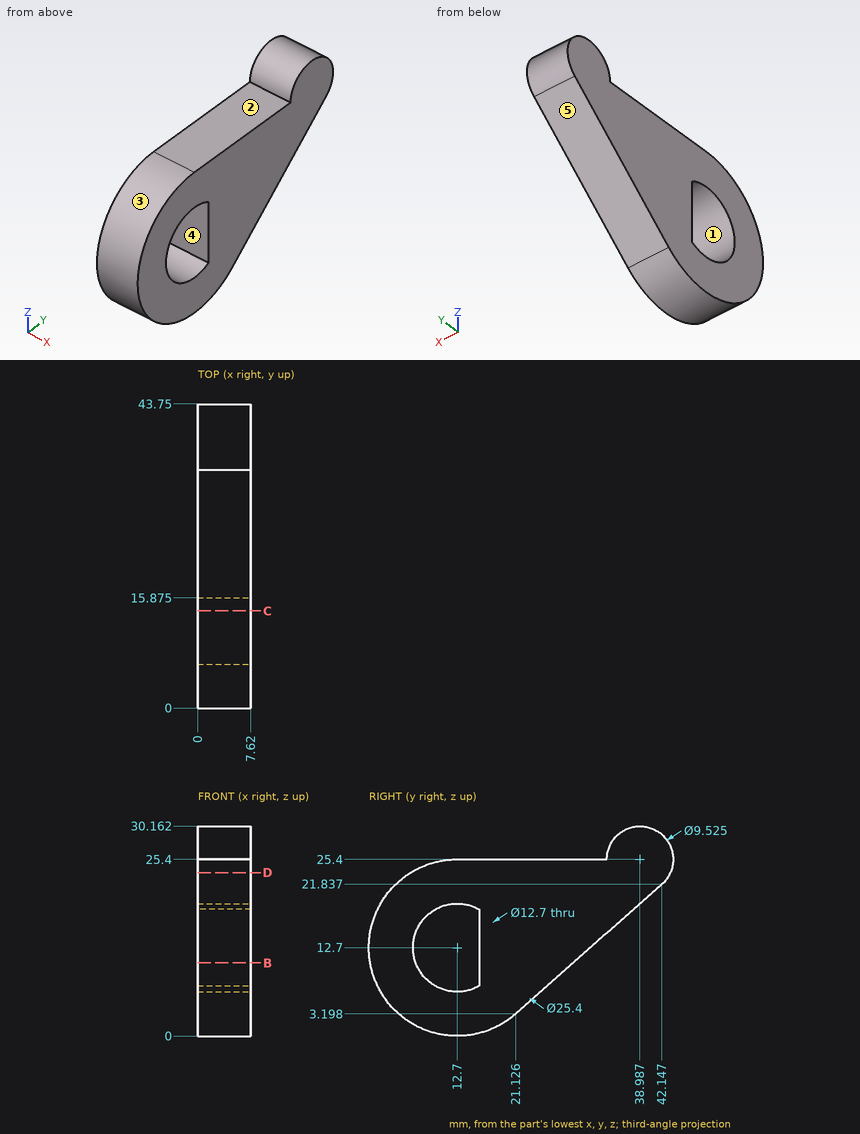
Part print with two shaded views. Sizes in mm from the minimum x, y, z corner. A direction names the side the tool comes from. Round coordinates to 2 decimals unless told otherwise and drop trailing zeros. Order: outer loops, then holes, each group sorted by start corner. A loop starts at its lowest first (then second) coordinate and runs counter-clockwise, first axis right, second up. Notation, with made-up numbers: (60.25, 78) - (80.25, 78) arc R28 ccw to (80.25, 98) - close; hole circle Ø10 at (55, -16). An arc over 180 degrees is marked (long way). Answer in a Markdown table with one row per item. Add a question column.
(1) Mould opens along Z. For the marked faces 3, 4 and 5 say: +Z half, -Z half, draft (parallel to the pull), parting line (faces both ways), or undercut.
(2) Band-saw the part on B-B on z = 10.5. List the corners of the cut face in (x, y) (1 decimal), and give its area (3 significant figures).
(3) Band-saw the part on C-C on y = 14. List the corners of the cut face in (x, z) (1 decimal).
(4) Band-saw the part on D-D on z = 23.5. List the corners of the cut face in (x, y) (1 decimal).
(5) 3-axis set-ups, long thin cutter, end or side, ignore diameter. For the marked faces 1 and 2: which of +Z, -Z, +X, -X, +Y, -Y reach the whole face in a straight line?
(6) Probe L1, parallel to Z at x = 2.5, y = 12.7; L2, parallel to Z at x = 4.5, y = 14 (1 decimal); L3, parallel to Y at x = 1.5, z = 13.5 (1 decimal). List the from-to ranges inside material, lowest first. Write a range as [from, to].
(7) Drop flat-ended pins along their axis: pin 1 Ø3 at (x, y) = (2, 19) entering from +Z; pin 2 Ø2 at (x, y) = (6, 6) entering from -Z. Give the stop position or say it passes through.
Data:
| question | item | result |
|---|---|---|
| 1 | face 3 | parting line |
| 1 | face 4 | undercut |
| 1 | face 5 | -Z half |
| 2 | outline | (0, 0.2) - (7.6, 0.2) - (7.6, 6.7) - (0, 6.7) - close; (0, 15.9) - (7.6, 15.9) - (7.6, 29.4) - (0, 29.4) - close |
| 2 | area | 153 mm^2 |
| 3 | outline | (0, 0.1) - (7.6, 0.1) - (7.6, 6.5) - (0, 6.5) - close; (0, 18.9) - (7.6, 18.9) - (7.6, 25.4) - (0, 25.4) - close |
| 4 | outline | (0, 6) - (7.6, 6) - (7.6, 43.4) - (0, 43.4) - close |
| 5 | face 1 | +X, -X |
| 5 | face 2 | +Z, +X, -X, -Y |
| 6 | L1 | z = [0, 6.35], [19.05, 25.4] |
| 6 | L2 | z = [0.1, 6.5], [18.9, 25.4] |
| 6 | L3 | y = [0, 6.4], [15.9, 32.7] |
| 7 | pin 1 | stops at z = 25.4 |
| 7 | pin 2 | stops at z = 1.35 |
